from build123d import *

# Parameters (mm, degrees)
SKETCH1_W                             = 42.418
SKETCH1_H                             = 20
BOSS_EXTRUDE1_DEPTH                   = 6.35
TAP_DRILL_FOR_M3X0_5_TAP2_D           = 2.5
TAP_DRILL_FOR_M3X0_5_TAP2_DEPTH       = 9.248924226
TAP_DRILL_FOR_M3X0_5_TAP2_CSINK_D     = 2.55
TAP_DRILL_FOR_M3X0_5_TAP2_CSINK_ANGLE = 90
TAP_DRILL_FOR_M3X0_5_TAP2_TIP         = 0.751075774
SKETCH12_W                            = 42.418
SKETCH12_H                            = 6.35
BOSS_EXTRUDE2_DEPTH                   = 6.35
SKETCH13_W                            = 42.418
SKETCH13_H                            = 6.35
BOSS_EXTRUDE3_DEPTH                   = 36.068
M3_CLEARANCE_HOLE1_D                  = 3.4
M3_CLEARANCE_HOLE1_CSINK_D            = 3.45
M3_CLEARANCE_HOLE1_CSINK_ANGLE        = 90
SKETCH17_W                            = 42.418
SKETCH17_H                            = 20
CUT_EXTRUDE1_DEPTH                    = 3.068
SKETCH19_R                            = 15
CUT_EXTRUDE2_DEPTH                    = 50.44739432


with BuildPart() as part:
    # Sketch1 → Boss-Extrude1 (new body)
    with BuildSketch(Plane(origin=(0, 0, 0), x_dir=(1, 0, 0), z_dir=(0, 1, 0))):
        Rectangle(SKETCH1_W, SKETCH1_H)
    extrude(amount=BOSS_EXTRUDE1_DEPTH)

    # Tap Drill for M3x0.5 Tap2
    with Locations(Plane(origin=(0, 0, 0), x_dir=(-1, 0, 0), z_dir=(0, -1, 0))):
        with Locations((-13.970620706, 6.587119009), (-13.970620706, -6.587119009), (13.970620706, 6.587119009), (13.970620706, -6.587119009)):
            CounterSinkHole(TAP_DRILL_FOR_M3X0_5_TAP2_D / 2, TAP_DRILL_FOR_M3X0_5_TAP2_CSINK_D / 2, depth=TAP_DRILL_FOR_M3X0_5_TAP2_DEPTH, counter_sink_angle=TAP_DRILL_FOR_M3X0_5_TAP2_CSINK_ANGLE)
            with Locations((0, 0, -(TAP_DRILL_FOR_M3X0_5_TAP2_DEPTH + TAP_DRILL_FOR_M3X0_5_TAP2_TIP / 2))):  # 118° drill point
                Cone(0, TAP_DRILL_FOR_M3X0_5_TAP2_D / 2, TAP_DRILL_FOR_M3X0_5_TAP2_TIP, mode=Mode.SUBTRACT)

    # Sketch12 → Boss-Extrude2 (add)
    with BuildSketch(Plane.XY.offset(10)):
        with Locations((0, 3.175)):
            Rectangle(SKETCH12_W, SKETCH12_H)
    extrude(amount=BOSS_EXTRUDE2_DEPTH)

    # Sketch13 → Boss-Extrude3 (add)
    with BuildSketch(Plane.XZ):
        with Locations((0, 13.175)):
            Rectangle(SKETCH13_W, SKETCH13_H)
    extrude(amount=BOSS_EXTRUDE3_DEPTH)

    # M3 Clearance Hole1 (through all)
    with Locations(Plane.XY.offset(16.35)):
        with Locations((-15.494, 0.635), (15.494, 0.635), (15.494, -30.353), (-15.494, -30.353)):
            CounterSinkHole(M3_CLEARANCE_HOLE1_D / 2, M3_CLEARANCE_HOLE1_CSINK_D / 2, counter_sink_angle=M3_CLEARANCE_HOLE1_CSINK_ANGLE)

    # Sketch17 → Cut-Extrude1 (cut)
    with BuildSketch(Plane.XZ):
        Rectangle(SKETCH17_W, SKETCH17_H)
    extrude(amount=-CUT_EXTRUDE1_DEPTH, mode=Mode.SUBTRACT)

    # Sketch19 → Cut-Extrude2 (cut, through all)
    with BuildSketch(Plane.XY.offset(16.35)):
        with Locations((0, -14.859)):
            Circle(SKETCH19_R)
    extrude(amount=-CUT_EXTRUDE2_DEPTH, mode=Mode.SUBTRACT)


solid = part.part
Work out the finished part from the listing and answer in its coordinate system (mm). Coordinates: 2 decimals unless noted, no trailing zeros. Loops run counter-clockwise (first coordinate to the right, second up) from the corner with the lowest first, then second, coordinate; pieces in that order, holes last. Notation, with made-up numbers: (-12, 26) -> (10, 26) arc R16 cw to (10, 40) -> close; hole circle Ø6 at (-39.5, -12). An arc over 180 degrees is marked (long way). Answer as CSV lines item,"result".
1) Flat-ended cylindrical pins translate along their axes: pin 1 (4 mm diameter, centred on x = -13.97, z = 6.59, fed in from +Y); pin 2 (4 mm diameter, centred on x = -7, y = 0, fed in from -Z); pin 3 (3 mm diameter, centred on x = -13.97, z = -6.59, fed in from -Y). Find the tip coordinate at first contact, or state that the pin passes through.
A:
pin 1,"stops at y = 6.35"
pin 2,"stops at z = 10"
pin 3,"stops at y = 3.07"
2) The part is cut by section B-B (z = 10.75). Give the vertices of the cut face in (x, y) (3 decimals).
A:
outline,"(-21.209, -36.068) -> (21.209, -36.068) -> (21.209, 6.35) -> (-21.209, 6.35) -> close; hole circle Ø3.4 at (-15.494, -30.353); hole circle Ø3.4 at (-15.494, 0.635); hole circle Ø30 at (0, -14.859); hole circle Ø3.4 at (15.494, -30.353); hole circle Ø3.4 at (15.494, 0.635)"
3) Straight lines are drawn through the part: probe 1 along X at (y, z) = (-30, 13.5); probe 2 along Z at (x, y) = (-16, -2); probe 3 along Y at (x, z) = (0, 14.25). For each, find the intervals that lie inside material, in ascending order.
A:
probe 1,"x = -21.21 to -17.16, -13.83 to 13.83, 17.16 to 21.21"
probe 2,"z = 10 to 16.35"
probe 3,"y = -36.07 to -29.86, 0.14 to 6.35"
4) The part is cut by section A-A (x = 0). Give the vertices of the cut face in (y, z).
A:
outline,"(-36.07, 10) -> (-29.86, 10) -> (-29.86, 16.35) -> (-36.07, 16.35) -> close; (0.14, 10) -> (3.07, 10) -> (3.07, -10) -> (6.35, -10) -> (6.35, 16.35) -> (0.14, 16.35) -> close"
5) For a pull along Y with two mould halves and no side action, classify faces 1 (the face through (0, 3.068, 0)), 2 (the face through (-13.796, 0.71, 13.118)), 3 (the face through (0, 5, -10)) as released by +Y, released by -Y, zero draft, split by the parting line, or undercut.
A:
face 1,"released by -Y"
face 2,"undercut"
face 3,"zero draft"
6) The part is cut by section C-C (y = -6). Give the vertices of the cut face in (x, z), and give its area (3 significant figures).
A:
outline,"(-21.21, 10) -> (-12.1, 10) -> (-12.1, 16.35) -> (-21.21, 16.35) -> close; (12.1, 10) -> (21.21, 10) -> (21.21, 16.35) -> (12.1, 16.35) -> close"
area,"116 mm²"
7) The part is cut by section D-D (x = 11.5). Give the vertices of the cut face in (y, z).
A:
outline,"(-36.07, 10) -> (-24.49, 10) -> (-24.49, 16.35) -> (-36.07, 16.35) -> close; (-5.23, 10) -> (3.07, 10) -> (3.07, -10) -> (6.35, -10) -> (6.35, 16.35) -> (-5.23, 16.35) -> close"
